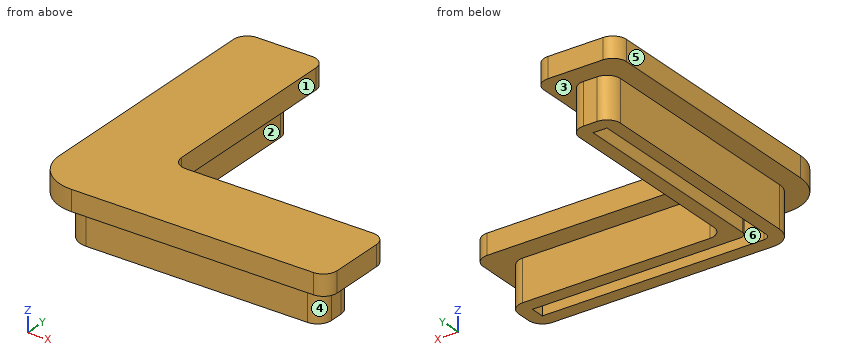
```python
from build123d import *

# Parameters (mm, degrees)
F1_DEPTH = 6
F3_DEPTH = 3
F4_R     = 2
F5_R     = 2


with BuildPart() as f1:
    # F0 (on Top) → F1 (new body)
    with BuildSketch(Plane.XY):
        with BuildLine():
            Line((-3, 34.2), (-3, 0))
            ThreePointArc((-3, 0), (-2.1213203436, -2.1213203436), (0, -3))
            Line((0, -3), (34.2, -3))
            Line((34.2, -3), (34.2, 3))
            Line((34.2, 3), (5, 3))
            ThreePointArc((5, 3), (3.5857864376, 3.5857864376), (3, 5))
            Line((3, 5), (3, 34.2))
            Line((3, 34.2), (-3, 34.2))
        make_face()
        with BuildLine():
            Line((1, 32.2), (1, 2))
            ThreePointArc((1, 2), (1.2928932188, 1.2928932188), (2, 1))
            Line((2, 1), (32.2, 1))
            Line((32.2, 1), (32.2, -1))
            Line((32.2, -1), (0, -1))
            ThreePointArc((0, -1), (-0.7071067812, -0.7071067812), (-1, 0))
            Line((-1, 0), (-1, 32.2))
            Line((-1, 32.2), (1, 32.2))
        make_face(mode=Mode.SUBTRACT)
    extrude(amount=F1_DEPTH)

    # F2 (on face) → F3 (join)
    with BuildSketch(Plane.XY.offset(6)):
        with BuildLine():
            Line((-6, 37.2), (-6, 0))
            ThreePointArc((-6, 0), (-4.2426406871, -4.2426406871), (0, -6))
            Line((0, -6), (37.2, -6))
            Line((37.2, -6), (37.2, 6))
            Line((37.2, 6), (6, 6))
            Line((6, 6), (6, 37.2))
            Line((6, 37.2), (-6, 37.2))
        make_face()
        with BuildLine():
            Line((-3, 0), (-3, 34.2))
            Line((-3, 34.2), (3, 34.2))
            Line((3, 34.2), (3, 5))
            ThreePointArc((3, 5), (3.5857864376, 3.5857864376), (5, 3))
            Line((5, 3), (34.2, 3))
            Line((34.2, 3), (34.2, -3))
            Line((34.2, -3), (0, -3))
            ThreePointArc((0, -3), (-2.1213203436, -2.1213203436), (-3, 0))
        make_face(mode=Mode.SUBTRACT)
        with BuildLine():
            Line((3, 34.2), (-3, 34.2))
            Line((-3, 34.2), (-3, 0))
            ThreePointArc((-3, 0), (-2.1213203436, -2.1213203436), (0, -3))
            Line((0, -3), (34.2, -3))
            Line((34.2, -3), (34.2, 3))
            Line((34.2, 3), (5, 3))
            ThreePointArc((5, 3), (3.5857864376, 3.5857864376), (3, 5))
            Line((3, 5), (3, 34.2))
        make_face()
        with BuildLine():
            ThreePointArc((0, -1), (-0.7071067812, -0.7071067812), (-1, 0))
            Line((-1, 0), (-1, 32.2))
            Line((-1, 32.2), (1, 32.2))
            Line((1, 32.2), (1, 2))
            ThreePointArc((1, 2), (1.2928932188, 1.2928932188), (2, 1))
            Line((2, 1), (32.2, 1))
            Line((32.2, 1), (32.2, -1))
            Line((32.2, -1), (0, -1))
        make_face(mode=Mode.SUBTRACT)
        with BuildLine():
            Line((-1, 32.2), (-1, 0))
            ThreePointArc((-1, 0), (-0.7071067812, -0.7071067812), (0, -1))
            Line((0, -1), (32.2, -1))
            Line((32.2, -1), (32.2, 1))
            Line((32.2, 1), (2, 1))
            ThreePointArc((2, 1), (1.2928932188, 1.2928932188), (1, 2))
            Line((1, 2), (1, 32.2))
            Line((1, 32.2), (-1, 32.2))
        make_face()
    extrude(amount=F3_DEPTH)

    # F4
    f4_edges = [f1.edges().sort_by_distance(p)[0] for p in [
        (6, 37.2, 7.5),
        (6, 6, 7.5),
        (37.2, 6, 7.5),
        (37.2, -6, 7.5),
        (-6, 37.2, 7.5),
    ]]
    fillet(f4_edges, radius=F4_R)

    # F5
    f5_edges = [f1.edges().sort_by_distance(p)[0] for p in [
        (-3, 34.2, 3),
        (3, 34.2, 3),
        (34.2, 3, 3),
        (34.2, -3, 3),
    ]]
    fillet(f5_edges, radius=F5_R)


solid = f1.part
```
Check sheet for the modelled part. Datum: model origin and axes. Units: mm. Face numbers are marked on the shaded views. A direction names the side the tool comes from. Coordinates: 2 decimals unless noted, no trailing zeros. Order: outer loops, then holes, each group sorted by start corner. A loop starts at its lowest first (then second) coordinate and runs counter-clockwise, first axis right, second up. Notation, with made-up numbers: M 31.5,-24 L 64.5,-24 A29 ccw 64.5,15 Z; hole C 76.25,72.5 d8. An arc over 180 degrees is marked long. Write each question's results on one line, items separated by ' | '. Start each with the question number.
1. Access from +Z, -Z, +X, -X, +Y, -Y to the whole of each face (thin tool, end or side, straight path). Record for the marked faces 1, 2 and 3.
2. Go/stop test with flat-tipped pins: P1, Ø3, axis at x = 17, z = 4, coming from the -Y side; P2, Ø3.5, axis at y = 16, z = 8, coming from the +X side; P3, Ø1.8, axis at x = 10.5, z = 1.5, coming from the +Y side. Record where each tip stops, or that it passes through.
3. Cross-section at A-A on z = 2.25. Record the cut outline in (x, y), and give its area (3 significant figures).
4. Cross-section at B-B on x = 19. Record the cut outline in (y, z), and give its area (3 significant figures).
5. Material ranges on probe 1 along X at (y, z) = (23.5, 0.5); probe 2 along Z at (x, y) = (4.5, 11), recorded low to high.
6. Mould release check, pull along Y, two halves, no side actions. Record for the marked faces 4, 5 and 6: +Y half, -Y half, draft (parallel to the pull), parting line (faces both ways), or undercut.
7. Cross-section at D-D on y = -1.5. Record the cut outline in (x, z), and give its area (3 significant figures).
Checks:
1) face 1: +Z, -Z, +X, +Y | face 2: -Z, +X, +Y | face 3: -Z
2) P1: stops at y = -3 | P2: stops at x = 6 | P3: stops at y = 3
3) outline: M -3,0 A3 ccw 0,-3 L 32.2,-3 A2 ccw 34.2,-1 L 34.2,1 A2 ccw 32.2,3 L 5,3 A2 cw 3,5 L 3,32.2 A2 ccw 1,34.2 L -1,34.2 A2 ccw -3,32.2 Z; hole M -1,0 A1 ccw 0,-1 L 32.2,-1 L 32.2,1 L 2,1 A1 cw 1,2 L 1,32.2 L -1,32.2 Z | area: 277 mm²
4) outline: M -6,6 L -3,6 L -3,0 L -1,0 L -1,6 L 1,6 L 1,0 L 3,0 L 3,6 L 6,6 L 6,9 L -6,9 Z | area: 60.0 mm²
5) probe 1: x = -3 to -1, 1 to 3 | probe 2: z = 6 to 9
6) face 4: -Y half | face 5: draft | face 6: undercut
7) outline: M -5.81,6 L -2.6,6 L -2.6,0 L 34.14,0 L 34.14,6 L 37.2,6 L 37.2,9 L -5.81,9 Z | area: 349 mm²
